Source: CAD feature listing. Evaluate the final solid. Frame: model axes, mm. A direction names the side the tool comes from. Give positions to 0.01 mm unless a question says otherwise; leave off trailing zeros. Loops run counter-clockwise (first coordinate to the right, second up) from the corner with the lowest first, then second, coordinate; pieces in that order, holes last.
from build123d import *

# Parameters (mm, degrees)
SKETCH1_W                    = 723.9
SKETCH1_H                    = 200.152
SKETCH1_R                    = 3.175
SKETCH1_R_2                  = 2.413
BASE_FLANGE1_DEPTH           = 1.6002
EDGE_FLANGE1_STRIP_W         = 7.874
EDGE_FLANGE1_STRIP_H         = 1.6002
EDGE_FLANGE1_STRIP_CUT_DEPTH = 723.9
EDGE_FLANGE1_DEPTH           = 723.9
SKETCH11_R                   = 19.05
CUT_EXTRUDE1_DEPTH           = 377.283721088
CUT_EXTRUDE3_REACH           = 378.388
SKETCH23_R                   = 5.55625
SKETCH23_R_2                 = 5.842
CUT_EXTRUDE4_REACH           = 378.388
SKETCH24_R                   = 4.445
EDGE_FLANGE2_DEPTH           = 197.8152
EDGE_FLANGE2_BEND_DEPTH      = 197.8152
SKETCH34_R                   = 3.175
CUT_EXTRUDE5_DEPTH           = 736.85314866
SKETCH35_R                   = 3.175
CUT_EXTRUDE6_DEPTH           = 379.53204476
CUT_EXTRUDE7_REACH           = 380.636
SKETCH36_R                   = 4.445


# Sheet-metal steps are written as plain solids
with BuildPart() as part:
    # Sketch1 → Base-Flange1 (new body)
    with BuildSketch(Plane(origin=(0, 0, 0), x_dir=(0, 0, -1), z_dir=(1, 0, 0))):
        Rectangle(SKETCH1_W, SKETCH1_H)
        with Locations((-207.518, -14.351)):
            Circle(SKETCH1_R, mode=Mode.SUBTRACT)
        with Locations((0, -17.526)):
            Circle(SKETCH1_R, mode=Mode.SUBTRACT)
        with Locations((207.518, -14.351)):
            Circle(SKETCH1_R, mode=Mode.SUBTRACT)
        with Locations((-104.638118017, 49.149)):
            Circle(SKETCH1_R_2, mode=Mode.SUBTRACT)
        with Locations((-104.638118017, -65.151)):
            Circle(SKETCH1_R_2, mode=Mode.SUBTRACT)
        with Locations((104.638118017, -65.151)):
            Circle(SKETCH1_R_2, mode=Mode.SUBTRACT)
        with Locations((104.638118017, 49.149)):
            Circle(SKETCH1_R_2, mode=Mode.SUBTRACT)
        with Locations((309.118, 49.149)):
            Circle(SKETCH1_R, mode=Mode.SUBTRACT)
        with Locations((309.118, -65.151)):
            Circle(SKETCH1_R, mode=Mode.SUBTRACT)
        with Locations((-309.118, -65.151)):
            Circle(SKETCH1_R_2, mode=Mode.SUBTRACT)
    extrude(amount=-BASE_FLANGE1_DEPTH)

    # Edge-Flange1 strip (across the edge) → Edge-Flange1 strip cut (cut)
    with BuildSketch(Plane(origin=(-1.6002, 100.076, 361.95), x_dir=(0, -1, 0), z_dir=(0, 0, -1))):
        with Locations((-1.6002, -0.8001)):
            Rectangle(EDGE_FLANGE1_STRIP_W, EDGE_FLANGE1_STRIP_H)
    extrude(amount=EDGE_FLANGE1_STRIP_CUT_DEPTH, mode=Mode.SUBTRACT)

    # Edge-Flange1 section (across the edge) → Edge-Flange1 (add)
    with BuildSketch(Plane(origin=(-1.6002, 100.076, 361.95), x_dir=(0, -1, 0), z_dir=(0, 0, -1))):
        with BuildLine():
            Line((0, 0.7366), (0, 23.7998))
            Line((0, 23.7998), (1.6002, 23.7998))
            Line((1.6002, 23.7998), (1.6002, 0.7366))
            ThreePointArc((1.6002, 0.7366), (1.815945145, 0.215745145), (2.3368, 0))
            Line((2.3368, 0), (2.3368, -1.6002))
            ThreePointArc((2.3368, -1.6002), (0.684432874, -0.915767126), (0, 0.7366))
        make_face()
    extrude(amount=EDGE_FLANGE1_DEPTH)

    # Sketch11 → Cut-Extrude1 (cut, through all)
    with BuildSketch(Plane.ZY.offset(1.6002)):
        with Locations((-174.498, -14.351)):
            Circle(SKETCH11_R)
        with Locations((33.02, -17.526)):
            Circle(SKETCH11_R)
        with Locations((174.498, -14.351)):
            Circle(SKETCH11_R)
    extrude(amount=-CUT_EXTRUDE1_DEPTH, mode=Mode.SUBTRACT)

    # Sketch23 → Cut-Extrude3 (cut, up to next)
    with BuildSketch(Plane(origin=(0, 0, 0), x_dir=(0, 0, -1), z_dir=(1, 0, 0)), mode=Mode.PRIVATE) as cut_extrude3_sk1:
        with Locations((-317.778063087, 62.003449438)):
            Circle(SKETCH23_R)
    cut_extrude3_tool1 = extrude(cut_extrude3_sk1.sketch, amount=-CUT_EXTRUDE3_REACH, mode=Mode.PRIVATE) & part.part
    # Sketch23 → Cut-Extrude3 (cut, up to next)
    with BuildSketch(Plane(origin=(0, 0, 0), x_dir=(0, 0, -1), z_dir=(1, 0, 0)), mode=Mode.PRIVATE) as cut_extrude3_sk2:
        with Locations((-320.548, 23.268449438)):
            Circle(SKETCH23_R_2)
    cut_extrude3_tool2 = extrude(cut_extrude3_sk2.sketch, amount=-CUT_EXTRUDE3_REACH, mode=Mode.PRIVATE) & part.part
    # Sketch23 → Cut-Extrude3 (cut, up to next)
    with BuildSketch(Plane(origin=(0, 0, 0), x_dir=(0, 0, -1), z_dir=(1, 0, 0)), mode=Mode.PRIVATE) as cut_extrude3_sk3:
        with Locations((-317.778063087, -15.466550562)):
            Circle(SKETCH23_R)
    cut_extrude3_tool3 = extrude(cut_extrude3_sk3.sketch, amount=-CUT_EXTRUDE3_REACH, mode=Mode.PRIVATE) & part.part
    add(cut_extrude3_tool1.solids().sort_by_distance((0, 62.003449, 317.778063))[0], mode=Mode.SUBTRACT)
    add(cut_extrude3_tool2.solids().sort_by_distance((0, 23.268449, 320.548))[0], mode=Mode.SUBTRACT)
    add(cut_extrude3_tool3.solids().sort_by_distance((0, -15.466551, 317.778063))[0], mode=Mode.SUBTRACT)

    # Sketch24 → Cut-Extrude4 (cut, up to next)
    with BuildSketch(Plane(origin=(0, 0, 0), x_dir=(0, 0, -1), z_dir=(1, 0, 0)), mode=Mode.PRIVATE) as cut_extrude4_sk1:
        with Locations((-338.860063087, 62.003449438)):
            Circle(SKETCH24_R)
    cut_extrude4_tool1 = extrude(cut_extrude4_sk1.sketch, amount=-CUT_EXTRUDE4_REACH, mode=Mode.PRIVATE) & part.part
    # Sketch24 → Cut-Extrude4 (cut, up to next)
    with BuildSketch(Plane(origin=(0, 0, 0), x_dir=(0, 0, -1), z_dir=(1, 0, 0)), mode=Mode.PRIVATE) as cut_extrude4_sk2:
        with Locations((-338.860063087, -15.466550562)):
            Circle(SKETCH24_R)
    cut_extrude4_tool2 = extrude(cut_extrude4_sk2.sketch, amount=-CUT_EXTRUDE4_REACH, mode=Mode.PRIVATE) & part.part
    add(cut_extrude4_tool1.solids().sort_by_distance((0, 62.003449, 338.860063))[0], mode=Mode.SUBTRACT)
    add(cut_extrude4_tool2.solids().sort_by_distance((0, -15.466551, 338.860063))[0], mode=Mode.SUBTRACT)

    # Edge-Flange2 section (across the edge) → Edge-Flange2 (add)
    with BuildSketch(Plane(origin=(-1.6002, 97.7392, -362.6866), x_dir=(0, 0, 1), z_dir=(0, -1, 0))):
        with BuildLine():
            Line((-1.6002, 0.7366), (-1.6002, 11.0998))
            Line((-1.6002, 11.0998), (0, 11.0998))
            Line((0, 11.0998), (0, 0.7366))
            ThreePointArc((0, 0.7366), (0.215745145, 0.215745145), (0.7366, 0))
            Line((0.7366, 0), (0.7366, -1.6002))
            ThreePointArc((0.7366, -1.6002), (-0.915767126, -0.915767126), (-1.6002, 0.7366))
        make_face()
    extrude(amount=EDGE_FLANGE2_DEPTH)

    # Edge-Flange2 section 2 (across the edge) → Edge-Flange2 bend (add)
    with BuildSketch(Plane(origin=(-1.6002, -100.076, 362.6866), x_dir=(0, 0, -1), z_dir=(0, 1, 0))):
        with BuildLine():
            Line((-1.6002, 0.7366), (-1.6002, 11.0998))
            Line((-1.6002, 11.0998), (0, 11.0998))
            Line((0, 11.0998), (0, 0.7366))
            ThreePointArc((0, 0.7366), (0.215745145, 0.215745145), (0.7366, 0))
            Line((0.7366, 0), (0.7366, -1.6002))
            ThreePointArc((0.7366, -1.6002), (-0.915767126, -0.915767126), (-1.6002, 0.7366))
        make_face()
    extrude(amount=EDGE_FLANGE2_BEND_DEPTH)

    # Sketch34 → Cut-Extrude5 (cut, through all)
    with BuildSketch(Plane.XY.offset(364.2868)):
        with Locations((-7.5184, 72.3392)):
            Circle(SKETCH34_R)
        with Locations((-7.5184, -1.1684)):
            Circle(SKETCH34_R)
        with Locations((-7.5184, -74.676)):
            Circle(SKETCH34_R)
    extrude(amount=-CUT_EXTRUDE5_DEPTH, mode=Mode.SUBTRACT)

    # Sketch35 → Cut-Extrude6 (cut, through all)
    with BuildSketch(Plane.ZY.offset(1.6002)):
        with Locations((349.25, 85.0392)):
            Circle(SKETCH35_R)
    extrude(amount=-CUT_EXTRUDE6_DEPTH, mode=Mode.SUBTRACT)

    # Sketch36 → Cut-Extrude7 (cut, up to next)
    with BuildSketch(Plane(origin=(0, 0, 0), x_dir=(0, 0, -1), z_dir=(1, 0, 0)), mode=Mode.PRIVATE) as cut_extrude7_sk1:
        with Locations((-249.960063087, 55.018449438)):
            Circle(SKETCH36_R)
    cut_extrude7_tool1 = extrude(cut_extrude7_sk1.sketch, amount=-CUT_EXTRUDE7_REACH, mode=Mode.PRIVATE) & part.part
    # Sketch36 → Cut-Extrude7 (cut, up to next)
    with BuildSketch(Plane(origin=(0, 0, 0), x_dir=(0, 0, -1), z_dir=(1, 0, 0)), mode=Mode.PRIVATE) as cut_extrude7_sk2:
        with Locations((-249.960063087, -8.481550562)):
            Circle(SKETCH36_R)
    cut_extrude7_tool2 = extrude(cut_extrude7_sk2.sketch, amount=-CUT_EXTRUDE7_REACH, mode=Mode.PRIVATE) & part.part
    add(cut_extrude7_tool1.solids().sort_by_distance((0, 55.018449, 249.960063))[0], mode=Mode.SUBTRACT)
    add(cut_extrude7_tool2.solids().sort_by_distance((0, -8.481551, 249.960063))[0], mode=Mode.SUBTRACT)


solid = part.part
1) Cut plane B-B (z = 291.5). Return loops of the section in (x, y).
Checks:
outline: (-25.4, 98.48) - (-2.34, 98.48) arc R0.74 cw to (-1.6, 97.74) - (-1.6, -100.08) - (0, -100.08) - (0, 97.74) arc R2.34 ccw to (-2.34, 100.08) - (-25.4, 100.08) - close
2) Reachability of faces 4 (the cylindrical face through (-0.789, 23.525, 326.384)), 5 (the flat face through (-14, 98.476, 5)), 6 (the flat face through (-1.6, 0, 5)) from +Z, -Z, +X, -X, +Y, -Y: full face, straight path, thin tool, end or side. Return the list, or none.
Checks:
face 4: +X, -X
face 5: +Z, -Z, -X, -Y
face 6: -X, -Y
3) Pull-direction query (Y, two-part tool) for faces 1 (the flat face through (-14, 100.076, 5)), 2 (the flat face through (-1, -100.076, -2)), 3 (the cylindrical face through (-0.81, -13.51, -193.53)); classes: released by +Y, released by -Y, zero draft, split by the parting line, or undercut.
Checks:
face 1: released by +Y
face 2: released by -Y
face 3: undercut
4) Ray query, probe 1 along Z at (x, y) = (-6, -32); probe 2 along X at (y, z) = (83, 32); probe 3 along Y at (x, z) = (-16.5, 314). Return the intervals inside material, ascending.
Checks:
probe 1: z = -364.29 to -362.69, 362.69 to 364.29
probe 2: x = -1.6 to 0
probe 3: y = 98.48 to 100.08
5) Cut plane C-C (x = -17). Return loops of the section in (y, z).
Checks:
outline: (98.48, -361.95) - (100.08, -361.95) - (100.08, 361.95) - (98.48, 361.95) - close
6) Contact query for flat-ended pins moving along their axis: P1, Ø7, axis at y = -15.47, z = 338.86, coming from the +X side; P2, Ø2.5, axis at x = -17.5, y = 98.5, coming from the -Z side; P3, Ø2, axis at y = 76.5, z = 258.5, coming from the -X side; P4, Ø4, axis at x = -6.5, z = -250, coming from the -Y side. Output: stop coordinate, or through.
Checks:
P1: passes through
P2: stops at z = -361.95
P3: stops at x = -1.6
P4: stops at y = 98.48
7) Cut plane A-A (z = 33.02). Return loops of the section in (x, y), and give its area (3 significant figures).
Checks:
outline: (-25.4, 98.48) - (-2.34, 98.48) arc R0.74 cw to (-1.6, 97.74) - (-1.6, 1.52) - (0, 1.52) - (0, 97.74) arc R2.34 ccw to (-2.34, 100.08) - (-25.4, 100.08) - close; (-1.6, -100.08) - (0, -100.08) - (0, -36.58) - (-1.6, -36.58) - close
area: 296 mm2
